from build123d import *

# Parameters (mm, degrees)
BOSS_EXTRUDE1_DEPTH = 6
BOSS_EXTRUDE2_START = -4
SKETCH2_W           = 9.735530135
SKETCH2_H           = 10.374223994
BOSS_EXTRUDE2_DEPTH = 8.5
SKETCH3_R           = 2.45
BOSS_EXTRUDE3_DEPTH = 7.5


with BuildPart() as part:
    # Sketch1 → Boss-Extrude1 (new, symmetric)
    with BuildSketch(Plane(origin=(0, 0, 0), x_dir=(0, 0, -1), z_dir=(1, 0, 0))):
        Polygon((-11.825, 6.5), (-11.825, 10.5), (11.825, 10.5), (11.825, 6.5), (16.125, 6.5), (16.125, 4.5), (11.825, 4.5), (11.825, -10.5), (-11.825, -10.5), (-11.825, 4.5), (-16.125, 4.5), (-16.125, 6.5), align=None)
    extrude(amount=BOSS_EXTRUDE1_DEPTH, both=True)

    # Sketch2 → Boss-Extrude2 (add)
    with BuildSketch(Plane(origin=(0, 10.5, 0), x_dir=(1, 0, 0), z_dir=(0, 1, 0)).offset(BOSS_EXTRUDE2_START)):
        with Locations((0.07225674, -4.853907597)):
            Rectangle(SKETCH2_W, SKETCH2_H)
    extrude(amount=BOSS_EXTRUDE2_DEPTH)

    # Sketch3 → Boss-Extrude3 (add)
    with BuildSketch(Plane(origin=(0, 10.5, 0), x_dir=(1, 0, 0), z_dir=(0, 1, 0))):
        with Locations(Location((0, -4.825, 0), (0, 0, 90))):
            Circle(SKETCH3_R)
    extrude(amount=BOSS_EXTRUDE3_DEPTH)


solid = part.part
Geometry: final body of the model. Coordinates: model frame, mm. A direction names the side the tool comes from. Give positions to 0.01 mm unless a question says otherwise; leave off trailing zeros. Loops run counter-clockwise (first coordinate to the right, second up) from the corner with the lowest first, then second, coordinate; pieces in that order, holes last. Notation, with made-up numbers: M 20,15.5 L 49,15.5 A21 ccw 49,19.5 Z; hole C 42,59.25 d8. An arc over 180 degrees is marked long. Put each result on its own line as item: value. Start each with the question number.
1) Ray query, line 1 along Z through (x, y) = (-1.75, 8.75) (3 decimals); line 2 along Y through (x, z) = (3, -1.5); line 3 along Y through (x, z) = (2, 8). Return the intervals inside material, ascending.
2) Cut plane A-A (z = 1). Output: boundary loops of the cut face in (x, y).
3) Cut plane C-C (y = 4). Output: boundary loops of the cut face in (x, z) (3 decimals), then the cut area to 3 significant figures.
4) Cut plane B-B (x = 0). Output: boundary loops of the cut face in (y, z) (3 decimals).
5) Cut plane D-D (x = -3.75). Output: boundary loops of the cut face in (y, z) (3 decimals), then the cut area to 3 significant figures.
6) Contact query for flat-ended pins moving along their axis: pin 1 (2 mm diameter, centred on x = 4, y = 3, fed in from +Z) (3 decimals); pin 2 (4.5 mm diameter, centred on x = -1, z = 13.5, fed in from +Y); pin 3 (5 mm diameter, centred on x = 0.5, y = 13.5, fed in from +Z). Output: stop coordinate, or through.
7) Access query for faces 1 (the flat face through (0, 6.5, 14)), 2 (the cylindrical face through (-0.108, 16.479, 7.273)), 3 (the flat face through (0, 6.5, -14)). Directions: +Z, -Z, +X, -X, +Y, -Y. A direction counts if a zero-diameter tool reaches every point of the face in a straight line with its end or side. Return the directions, or none.
Verdict:
1. line 1: -11.825 to 11.825
1. line 2: -10.5 to 10.5
1. line 3: -10.5 to 15
2. outline: M -6,-10.5 L 6,-10.5 L 6,10.5 L 4.94,10.5 L 4.94,15 L -4.8,15 L -4.8,10.5 L -6,10.5 Z
3. outline: M -6,-11.825 L 6,-11.825 L 6,11.825 L -6,11.825 Z
3. area: 284 mm2
4. outline: M -10.5,-11.825 L 4.5,-11.825 L 4.5,-16.125 L 6.5,-16.125 L 6.5,-11.825 L 10.5,-11.825 L 10.5,-0.333 L 15,-0.333 L 15,2.375 L 18,2.375 L 18,7.275 L 15,7.275 L 15,10.041 L 10.5,10.041 L 10.5,11.825 L 6.5,11.825 L 6.5,16.125 L 4.5,16.125 L 4.5,11.825 L -10.5,11.825 Z
5. outline: M -10.5,-11.825 L 4.5,-11.825 L 4.5,-16.125 L 6.5,-16.125 L 6.5,-11.825 L 10.5,-11.825 L 10.5,-0.333 L 15,-0.333 L 15,10.041 L 10.5,10.041 L 10.5,11.825 L 6.5,11.825 L 6.5,16.125 L 4.5,16.125 L 4.5,11.825 L -10.5,11.825 Z
5. area: 561 mm2
6. pin 1: z = 11.825
6. pin 2: y = 10.5
6. pin 3: z = 10.04
7. face 1: +Z, +X, -X, +Y
7. face 2: +Y
7. face 3: -Z, +X, -X, +Y
